Check sheet for the modelled part. Datum: model origin and axes. Units: mm. A direction names the side the tool comes from. Give positions to 0.01 mm unless a question says otherwise; leave off trailing zeros. Order: outer loops, then holes, each group sorted by start corner. A loop starts at its lowest first (then second) coordinate and runs counter-clockwise, first axis right, second up.
```python
from build123d import *

# Parameters (mm, degrees)
EXTRUDE_BODY_DEPTH = 10
SKETCH2_W          = 1.9
SKETCH2_H          = 0.9
CUT_EXTRUDE1_DEPTH = 12.703418304
SKETCH3_W          = 1.9
SKETCH3_H          = 0.9
CUT_EXTRUDE2_DEPTH = 12.703418304
CUT_EXTRUDE3_DEPTH = 12.703418304
HOLE_REVOLVE_D     = 5
EDGE_FILLETS_R     = 0.2


with BuildPart() as part:
    # Sketch1 → Extrude Body (new body)
    with BuildSketch(Plane.XY.offset(5)):
        Polygon((4.9, -1), (4.9, 0.9), (-4.9, 0.9), (-4.9, -1), (-2.3, -3.6), (2.3, -3.6), align=None)
    extrude(amount=-EXTRUDE_BODY_DEPTH)

    # Sketch2 → Cut-Extrude1 (cut, through all)
    with BuildSketch(Plane(origin=(0, 0, -5), x_dir=(-1, 0, 0), z_dir=(0, 0, -1))):
        with Locations((3.95, 0.45)):
            Rectangle(SKETCH2_W, SKETCH2_H)
    extrude(amount=-CUT_EXTRUDE1_DEPTH, mode=Mode.SUBTRACT)

    # Sketch3 → Cut-Extrude2 (cut, through all)
    with BuildSketch(Plane(origin=(0, 0, -5), x_dir=(-1, 0, 0), z_dir=(0, 0, -1))):
        with Locations((-3.95, 0.45)):
            Rectangle(SKETCH3_W, SKETCH3_H)
    extrude(amount=-CUT_EXTRUDE2_DEPTH, mode=Mode.SUBTRACT)

    # Sketch4 → Cut-Extrude3 (cut, through all)
    with BuildSketch(Plane(origin=(0, 0, -5), x_dir=(-1, 0, 0), z_dir=(0, 0, -1))):
        Polygon((0.4, 0.9), (-0.4, 0.9), (0, 0.5), align=None)
    extrude(amount=-CUT_EXTRUDE3_DEPTH, mode=Mode.SUBTRACT)

    # Hole Revolve (through all)
    with Locations(Plane(origin=(0, -3.6, 0), x_dir=(-1, 0, 0), z_dir=(0, -1, 0))):
        with Locations((0, 0)):
            Hole(HOLE_REVOLVE_D / 2)

    # Edge Fillets
    edge_fillets_edges = [part.edges().sort_by_distance(p)[0] for p in [
        (4.9, 0, 0),
        (3, 0, 0),
        (-4.9, -1, 0),
        (3, 0.9, 0),
        (-3, 0, 0),
        (0.4, 0.9, -3.733896268),
        (0, 0.5, 3.75),
        (-0.4, 0.9, -3.733896268),
        (4.9, -1, 0),
        (-3, 0.9, 0),
        (0, 0.5, -3.75),
        (-0.4, 0.9, 3.733896268),
        (-4.9, 0, 0),
        (-2.3, -3.6, -2.989897949),
        (0.4, 0.9, 3.733896268),
        (2.3, -3.6, -2.989897949),
    ]]
    fillet(edge_fillets_edges, radius=EDGE_FILLETS_R)


solid = part.part
```
Q1. Sectioned sample at A-A, the plane z = 1.5. Record the cut outline in (x, y).
Q2. Sectioned sample at D-D, the plane z = 0. Record the cut outline in (x, y).
Q3. Tool access check on faces 1 (the flat face through (0, -3.6, 3)), 2 (the flat face through (4, 0, 0)), 3 (the flat face through (-4, 0, 0)). Record the directions out of +Z, -Z, +X, -X, +Y, -Y that give a thin tool (end or side, any length) a straight path to the whole face; none if there is none.
Q4. Draft check along Z on faces 4 (the flat face through (0, -1, 5)), 5 (the cylindrical face through (-0.54, -1.32, 2.44)), 6 (the flat face through (3.6, -2.3, 0.1)). Enter one of: pulls with the +Z half, pulls with the -Z half, needs draft (parallel to the pull), parting line crosses it, or undercut.
Q5. Sectioned sample at B-B, the plane x = 0. Record the cut outline in (y, z), plus the area to 3 significant figures.
Q6. Go/stop test with a flat-tipped pin: P1, Ø4, axis at x = 3.5, z = 3.5, coming from the -Y side. Record where the tip stops, or that it passes through.
Q7. Sectioned sample at C-C, the plane y = -1.35. Record the cut outline in (x, z).
Q8. Material ranges on line 1 (Z direction, x = -0.5, y = 0.15); line 2 (Z direction, x = 0, y = -0.1); line 3 (X direction, y = -0.8, z = -0.5), recorded low to high.
Filled in:
1. outline: (-4.9, -0.92) arc R0.2 ccw to (-4.84, -1.06) - (-2.3, -3.6) - (-2, -3.6) - (-2, 0.9) - (-2.8, 0.9) arc R0.2 ccw to (-3, 0.7) - (-3, 0.2) arc R0.2 cw to (-3.2, 0) - (-4.7, 0) arc R0.2 ccw to (-4.9, -0.2) - close; (2, -3.6) - (2.3, -3.6) - (4.84, -1.06) arc R0.2 ccw to (4.9, -0.92) - (4.9, -0.2) arc R0.2 ccw to (4.7, 0) - (3.2, 0) arc R0.2 cw to (3, 0.2) - (3, 0.7) arc R0.2 ccw to (2.8, 0.9) - (2, 0.9) - close
2. outline: (-4.9, -0.92) arc R0.2 ccw to (-4.84, -1.06) - (-2.5, -3.4) - (-2.5, 0.9) - (-2.8, 0.9) arc R0.2 ccw to (-3, 0.7) - (-3, 0.2) arc R0.2 cw to (-3.2, 0) - (-4.7, 0) arc R0.2 ccw to (-4.9, -0.2) - close; (2.5, -3.4) - (4.84, -1.06) arc R0.2 ccw to (4.9, -0.92) - (4.9, -0.2) arc R0.2 ccw to (4.7, 0) - (3.2, 0) arc R0.2 cw to (3, 0.2) - (3, 0.7) arc R0.2 ccw to (2.8, 0.9) - (2.5, 0.9) - close
3. face 1: +Z, -Z, +X, -X, -Y
3. face 2: +Z, -Z, +X, +Y
3. face 3: +Z, -Z, -X, +Y
4. face 4: pulls with the +Z half
4. face 5: undercut
4. face 6: needs draft
5. outline: (-3.6, -5) - (0.58, -5) - (0.58, -2.5) - (-3.6, -2.5) - close; (-3.6, 2.5) - (0.58, 2.5) - (0.58, 5) - (-3.6, 5) - close
5. area: 20.9 mm2
6. P1: stops at y = -3.6
7. outline: (-4.55, -5) - (4.55, -5) - (4.55, 5) - (-4.55, 5) - close; hole circle Ø5 at (0, 0)
8. line 1: z = -5 to -2.45, 2.45 to 5
8. line 2: z = -5 to -2.5, 2.5 to 5
8. line 3: x = -4.9 to -2.45, 2.45 to 4.9
